Could you check a few things on this model? Use its own coordinates, in mm. A direction names the side the tool comes from. Give positions to 0.01 mm unless a question says otherwise; leave off trailing zeros. Loops run counter-clockwise (first coordinate to the right, second up) from the corner with the lowest first, then second, coordinate; pieces in that order, holes last. Notation, with made-up numbers: (-26.5, 82.5) - (-18.5, 82.5) arc R21 ccw to (-18.5, 121.5) - close; hole circle Ø1 at (15.25, 15.5). An arc over 180 degrees is marked (long way). One line per item, written item: value. Start each with the question number.
Q1. I want a section at A-A (z = 14). Please give me the cut outline in (x, y).
Q2. I want a section at C-C (x = -15.5). Please give me the cut outline in (y, z).
Q3. If I drill on line 1 (Y direction, x = -5, z = 15.5); line 2 (Y direction, x = -23.5, z = 79.5); line 3 (X direction, y = -59, z = 7.5), over which ranges is the centre line in solid material (lowest first)? Write a range as from..to.
Q4. I want a section at B-B (y = -69). Please give me the cut outline in (x, z).
Q5. For faces 1 (the face through (0, -29, 0)), 2 (the face through (0, -17, 67)), 3 (the face through (0, -15, 13)), which set-ups out of +Z, -Z, +X, -X, +Y, -Y let a thin tool reach every point of the face, with its end or its side?
Q6. I want a section at D-D (z = 38.5). Please give me the cut outline in (x, y).
Q7. If we mould it in two halves opening along X, with no side actions, what happens to faces 4 (the face through (0, 0, 2)), 5 (the face through (-2, -75, 110)), 6 (the face through (29.5, -40, 54))? For each: released by +X, released by -X, zero draft, split by the parting line, or undercut.
Q8. I'm going to push flat-ended pins straight in: P1, Ø11, axis at x = -13, y = 0.5, coming from the +Z side; P2, Ø16.5, axis at x = 8.5, z = 40, coming from the +Y side. Where does each tip first touch, or does it pass through?
```python
from build123d import *

# Parameters (mm, degrees)
SKETCH_W       = 59
SKETCH_H       = 34
PAD_DEPTH      = 25
THICKNESS_T    = -2
SKETCH002_W    = 59
SKETCH002_H    = 59
PAD001_DEPTH   = 110
THICKNESS001_T = -2
FILLET_R       = 2
FILLET001_R    = 2
POCKET_DEPTH   = 2


with BuildPart() as body:
    # Sketch → Pad (new body)
    with BuildSketch(Plane.XY):
        Rectangle(SKETCH_W, SKETCH_H)
    extrude(amount=PAD_DEPTH)

    # Thickness
    thickness_openings = [body.faces().sort_by_distance(p)[0] for p in [
        (0, 0, 25),
    ]]
    offset(amount=THICKNESS_T, openings=thickness_openings)


with BuildPart() as body001:
    # Sketch002 → Pad001 (new body)
    with BuildSketch(Plane.XY):
        with Locations((0, -46.5)):
            Rectangle(SKETCH002_W, SKETCH002_H)
    extrude(amount=PAD001_DEPTH)

    # Thickness001
    thickness001_openings = [body001.faces().sort_by_distance(p)[0] for p in [
        (0, -46.5, 110),
    ]]
    offset(amount=THICKNESS001_T, openings=thickness001_openings)

    # Boolean: union Body
    add(body.part)

    # Fillet
    fillet_edges = [body001.edges().sort_by_distance(p)[0] for p in [
        (29.5, -76, 55),
        (29.5, 17, 12.5),
        (-29.5, -76, 55),
        (-29.5, 17, 12.5),
    ]]
    fillet(fillet_edges, radius=FILLET_R)

    # Fillet001
    fillet001_edges = [body001.edges().sort_by_distance(p)[0] for p in [
        (29.5, -17, 67.5),
        (-29.5, -17, 67.5),
    ]]
    fillet(fillet001_edges, radius=FILLET001_R)

    # Sketch003 → Pocket (cut)
    with BuildSketch(Plane(origin=(0, -17, 0), x_dir=(-1, 0, 0), z_dir=(0, 1, 0))):
        with BuildLine():
            add(Edge.make_bspline(
                [(0, 75.6251), (-2.511254, 80.679903), (-7.485486, 83.314581), (-11.174629, 85.509438), (-13.605908, 89.797189), (-13.37285, 93.451754), (-11.541057, 97.022131), (-7.614382, 99.161534), (-3.819055, 99.187138), (-1.554081, 97.750555), (0, 95.2257)],
                knots=[0, 0, 0, 0, 0.125, 0.25, 0.375, 0.5, 0.625, 0.75, 0.875, 1, 1, 1, 1], degree=3))
            add(Edge.make_bspline(
                [(0, 75.6251), (2.511254, 80.679903), (7.485486, 83.314581), (11.174629, 85.509438), (13.605908, 89.797189), (13.37285, 93.451754), (11.541057, 97.022131), (7.614382, 99.161534), (3.819055, 99.187138), (1.554081, 97.750555), (0, 95.2257)],
                knots=[0, 0, 0, 0, 0.125, 0.25, 0.375, 0.5, 0.625, 0.75, 0.875, 1, 1, 1, 1], degree=3))
        make_face()
    extrude(amount=-POCKET_DEPTH, mode=Mode.SUBTRACT)


solid = body001.part
```
Worked answers:
1. outline: (-29.5, -74) arc R2 ccw to (-27.5, -76) - (27.5, -76) arc R2 ccw to (29.5, -74) - (29.5, 15) arc R2 ccw to (27.5, 17) - (-27.5, 17) arc R2 ccw to (-29.5, 15) - close; hole (-27.5, -74) - (27.5, -74) - (27.5, -19) - (-27.5, -19) - close; hole (-27.5, -15) - (27.5, -15) - (27.5, 15) - (-27.5, 15) - close
2. outline: (-76, 0) - (17, 0) - (17, 25) - (15, 25) - (15, 2) - (-15, 2) - (-15, 25) - (-17, 25) - (-17, 110) - (-19, 110) - (-19, 2) - (-74, 2) - (-74, 110) - (-76, 110) - close
3. line 1: y = -76..-74, -19..-15, 15..17
3. line 2: y = -76..-74, -19..-17
3. line 3: x = -29.5..-27.5, 27.5..29.5
4. outline: (-29.5, 0) - (29.5, 0) - (29.5, 110) - (27.5, 110) - (27.5, 2) - (-27.5, 2) - (-27.5, 110) - (-29.5, 110) - close
5. face 1: -Z, +X, -X, +Y, -Y
5. face 2: +Z, +X, -X, +Y
5. face 3: +Z
6. outline: (-29.5, -74) arc R2 ccw to (-27.5, -76) - (27.5, -76) arc R2 ccw to (29.5, -74) - (29.5, -19) arc R2 ccw to (27.5, -17) - (-27.5, -17) arc R2 ccw to (-29.5, -19) - close; hole (-27.5, -74) - (27.5, -74) - (27.5, -19) - (-27.5, -19) - close
7. face 4: undercut
7. face 5: zero draft
7. face 6: released by +X
8. P1: stops at z = 2
8. P2: stops at y = -17
